For this review, take the finished solid that the model builds, in its own axes (mm). Coordinates: 2 decimals unless noted, no trailing zeros. Loops run counter-clockwise (first coordinate to the right, second up) from the corner with the lowest first, then second, coordinate; pieces in that order, holes last.
1. Take a section at A-A, the plane x = -60.5. State the section outline as (y, z) points.
2. Take a section at C-C, the plane y = -2. Count the separate pieces of the cut face and the enclosed holes in it, then the cut area to 3 significant figures.
3. Take a section at D-D, the plane x = 0. State the section outline as (y, z) points, then the cut area to 3 significant figures.
4. To check wall thickness, follow probe 1 along Z at (x, y) = (-72, 0.75); probe 2 along X at (y, z) = (-2.15, -5); probe 3 along X at (y, z) = (-0.25, -88.5). State the ranges of each line that lie inside material, in increasing order.
5. Take a section at B-B, the plane z = -34.5. State the section outline as (x, y) points, then the cut area to 3 significant figures.
6. Clearance check with flat-ended pins moving along their axes: P1, Ø2, axis at x = -24, y = -1, coming from the +Z side; P2, Ø5.5, axis at x = 90, z = 55, coming from the +Y side; P3, Ø5, axis at x = 20, z = -90, coming from the -Y side; P4, Ø1, axis at y = -2, z = 83.5, coming from the -X side. State where each tip first meets the part, or that it passes through.
```python
from build123d import *

# Parameters (mm, degrees)
SKETCH_1_R               = 3
SKETCH_1_R_2             = 2.1
EXTRUDE_1_DEPTH          = 3
CHAMFER_1_SIZE           = 2
CHAMFER_3_SIZE           = 4
CUT_EXTRUDE_1_DEPTH      = 146.124084838
CHAMFER_4_SIZE           = 3
CUT_EXTRUDE_2_DEPTH      = 146.124084838
PATTERN_CIRCULAR_1_COUNT = 3


with BuildPart() as part:
    # 草图1 → 凸台-拉伸1 (new, symmetric)
    with BuildSketch(Plane(origin=(0, 0, 0), x_dir=(1, 0, 0), z_dir=(0, 1, 0))):
        Polygon((-50, 100), (50, 100), (100, -45), (100, -105), (80, -105), (-100, -5), (-100, 55), align=None)
        with Locations(Location((0, 0, 0), (0, 0, 270))):
            Circle(SKETCH_1_R, mode=Mode.SUBTRACT)
        with Locations(Location((-20, 90, 0), (0, 0, 270))):
            Circle(SKETCH_1_R_2, mode=Mode.SUBTRACT)
        with Locations(Location((-90, 45, 0), (0, 0, 270))):
            Circle(SKETCH_1_R_2, mode=Mode.SUBTRACT)
        with Locations(Location((-90, 5, 0), (0, 0, 270))):
            Circle(SKETCH_1_R_2, mode=Mode.SUBTRACT)
        with Locations(Location((20, 90, 0), (0, 0, 90))):
            Circle(SKETCH_1_R_2, mode=Mode.SUBTRACT)
        with Locations(Location((90, -55, 0), (0, 0, 270))):
            Circle(SKETCH_1_R_2, mode=Mode.SUBTRACT)
        with Locations(Location((90, -95, 0), (0, 0, 270))):
            Circle(SKETCH_1_R_2, mode=Mode.SUBTRACT)
    extrude(amount=EXTRUDE_1_DEPTH, both=True)

    # 倒角1
    chamfer_1_edges = [part.edges().sort_by_distance(p)[0] for p in [
        (-20, 3, -92.1),
        (-90, 3, -47.1),
        (-90, 3, -7.1),
        (90, 3, 52.9),
        (90, 3, 92.9),
        (20, 3, -87.9),
    ]]
    chamfer(chamfer_1_edges, length=CHAMFER_1_SIZE)

    # 倒角3
    chamfer_3_edges = [part.edges().sort_by_distance(p)[0] for p in [
        (100, 0, 105),
    ]]
    chamfer(chamfer_3_edges, length=CHAMFER_3_SIZE)

    # 草图2 → 切除-拉伸1 (cut, through all)
    with BuildSketch(Plane(origin=(0, 3, 0), x_dir=(1, 0, 0), z_dir=(0, 1, 0))):
        with BuildLine():
            Line((-78.344823658, 54.309222637), (-51.225659109, 78.716470731))
            ThreePointArc((-51.225659109, 78.716470731), (-44.16436472, 78.344823658), (-44.536011793, 71.283529269))
            Line((-44.536011793, 71.283529269), (-71.655176342, 46.876281175))
            ThreePointArc((-71.655176342, 46.876281175), (-78.716470731, 47.247928248), (-78.344823658, 54.309222637))
        make_face()
        with BuildLine():
            Line((70.669187988, -36.629953417), (32.738153505, 73.370046583))
            ThreePointArc((32.738153505, 73.370046583), (35.835064997, 79.726864908), (42.191883322, 76.629953417))
            Line((42.191883322, 76.629953417), (80.122917804, -33.370046583))
            ThreePointArc((80.122917804, -33.370046583), (77.026006313, -39.726864908), (70.669187988, -36.629953417))
        make_face()
        with BuildLine():
            Line((67.571785344, -80.936052734), (-72.428214656, -3.158274956))
            ThreePointArc((-72.428214656, -3.158274956), (-74.370786381, 3.64072608), (-67.571785344, 5.583297805))
            Line((-67.571785344, 5.583297805), (72.428214656, -72.194479973))
            ThreePointArc((72.428214656, -72.194479973), (74.370786381, -78.993481009), (67.571785344, -80.936052734))
        make_face()
    extrude(amount=-CUT_EXTRUDE_1_DEPTH, mode=Mode.SUBTRACT)

    # 倒角4
    chamfer_4_edges = [part.edges().sort_by_distance(p)[0] for p in [
        (0, 3, -3),
    ]]
    chamfer(chamfer_4_edges, length=CHAMFER_4_SIZE)

    # 草图3 → 切除-拉伸2 (cut, through all)
    with BuildSketch(Plane(origin=(0, 3, 0), x_dir=(1, 0, 0), z_dir=(0, 1, 0))):
        with BuildLine():
            ThreePointArc((20.541451993, 20.541451993), (16.662395476, 23.796366887), (12.277060504, 26.328241213))
            ThreePointArc((12.277060504, 26.328241213), (6.894910006, 24.369298636), (8.853852583, 18.987148138))
            ThreePointArc((8.853852583, 18.987148138), (12.016426342, 17.161235328), (14.813887066, 14.813887066))
            ThreePointArc((14.813887066, 14.813887066), (20.541451993, 14.813887066), (20.541451993, 20.541451993))
        make_face()
    cut_extrude_2 = extrude(amount=-CUT_EXTRUDE_2_DEPTH, mode=Mode.SUBTRACT)

    # 阵列(圆周)1: 切除-拉伸2 ×3 about axis
    pattern_circular_1_axis = Axis((0, 0, 0), (0, 1, 0))
    for i in range(1, PATTERN_CIRCULAR_1_COUNT):
        add(cut_extrude_2.rotate(pattern_circular_1_axis, i * 360 / PATTERN_CIRCULAR_1_COUNT), mode=Mode.SUBTRACT)


solid = part.part
```
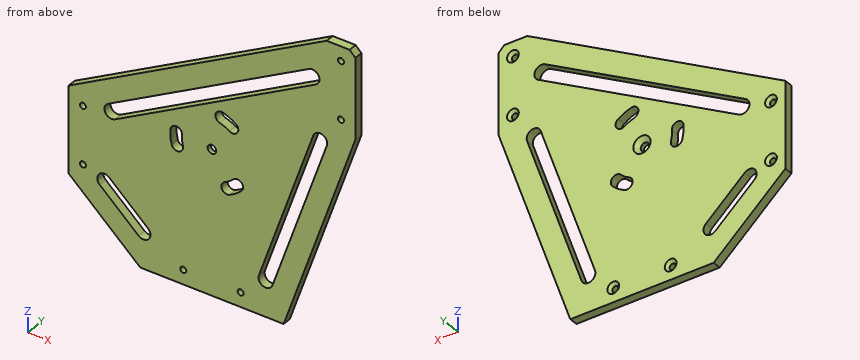
Results list:
1. outline: (-3, -90.55) - (3, -90.55) - (3, -70.37) - (-3, -70.37) - close; (-3, -56.92) - (3, -56.92) - (3, -1.65) - (-3, -1.65) - close; (-3, 9.79) - (3, 9.79) - (3, 26.94) - (-3, 26.94) - close
2. separate pieces: 1
2. enclosed holes: 13
2. area: 23,400 mm2
3. outline: (-3, -100) - (3, -100) - (3, -6) - (0, -3) - (-3, -3) - close; (-3, 3) - (0, 3) - (3, 6) - (3, 31.96) - (-3, 31.96) - close; (-3, 43.4) - (3, 43.4) - (3, 60.56) - (-3, 60.56) - close
3. area: 850 mm2
4. probe 1: z = -80.2 to -60.02, -46.59 to -5.8, 3.4 to 20.56
4. probe 2: x = -100 to -92.1, -87.9 to -73.26, -66.52 to -28.62, -20.34 to 56.31, 66.89 to 82.76
4. probe 3: x = -62.78 to -21.47, -18.53 to 18.53, 21.47 to 53.97
5. outline: (-100, -3) - (46.14, -3) - (46.14, 3) - (-100, 3) - close; (56.72, -3) - (72.59, -3) - (72.59, 3) - (56.72, 3) - close
5. area: 972 mm2
6. P1: stops at z = 47.78
6. P2: stops at y = 1.65
6. P3: stops at y = -3
6. P4: stops at x = 40.4
